Autodesk Inventor part; units mm, degrees
ref_plane "РабПлоскость1" through (-7.5, 3, -10) normal (0, 0, -1) x (-1, 0, 0)
ref_plane "YZ Plane" through (0, 0, 0) normal (1, 0, 0) x (0, 1, 0)
ref_plane "XZ Plane" through (0, 0, 0) normal (0, 1, 0) x (-1, 0, 0)
sketch "Эскиз1" plane through (0, 0, 0) normal (0, 1, 0) x (-1, 0, 0)
  line L0 (-7.5, 14.5) -> (7.5, 14.5)
  line L1 (7.5, 14.5) -> (7.5, -14.5)
  line L2 (7.5, -14.5) -> (-7.5, -14.5)
  line L3 (-7.5, -14.5) -> (-7.5, 14.5)
  line L4 (-7.5, 14.5) -> (7.5, -14.5) construction
  line L5 (7.5, 14.5) -> (-7.5, -14.5) construction
  point P0 (0, 0)
  dimension "d0" = 15
  dimension "d1" = 29
extrude "Выдавливание1" add sketch "Эскиз1" along normal blind 27
sketch "Эскиз2" plane through (0, 0, 0) normal (0, -1, 0) x (1, 0, 0)
  line L0 (12.5, 19.5) -> (-12.5, 19.5)
  line L1 (-12.5, 19.5) -> (-12.5, -15.5)
  line L2 (-12.5, -15.5) -> (12.5, -15.5)
  line L3 (12.5, -15.5) -> (12.5, 19.5)
  line L4 (7.5, 14.5) -> (7.5, -14.5)
  line L5 (-7.5, 14.5) -> (7.5, 14.5)
  point P0 (0, 0)
  dimension "d4" = 25
  dimension "d5" = 35
  dimension "d6" = 5
  dimension "d7" = 5
extrude "Выдавливание2" add sketch "Эскиз2" along normal blind 3.5
fillet "Сопряжение1" radius 1 1 edges at (-12.5, -1.75, 19.5)
fillet "Сопряжение2" radius 1 2 edges at (12.5, -1.75, 19.5) (12.5, -1.75, -15.5)
fillet "Сопряжение3" radius 1 1 edges at (-12.5, -1.75, -15.5)
sketch "Эскиз3" plane through (7.5, 27, 14.5) normal (1, 0, 0) x (0, 0, -1)
  line L0 (14.2, 0) -> (14.2, -20.2)
  line L1 (0, -27) -> (0, 0)
  line L2 (0, 0) -> (29, 0)
  line L3 (29, -27) -> (-4, -27)
  line L4 (-4, -27) -> (29, -27)
  line L5 (18.4, -27) -> (18.4, -24)
  line L6 (18.4, -24) -> (29, -24)
  line L7 (29, -27) -> (29, 0)
  line L8 (29, 0) -> (0, 0)
  line L9 (19.6, 0) -> (19.6, -15.6)
  line L10 (19.6, -15.6) -> (29, -21.4)
  line L11 (0, -25.2) -> (9.2, -25.2)
  line L12 (9.2, -25.2) -> (14.2, -20.2)
  point P0 (14.5, -27)
  dimension "d17" = 3
  dimension "d18" = 9.4
  dimension "d43" = 5
extrude "Выдавливание3" cut sketch "Эскиз3" against normal blind 23 contours L0 L12 L11 L1 L2 | L2 L7 L10 L9 | L5 L6 L7 L3
sketch "Эскиз5" plane through (0, 27, 0) normal (0, 1, 0) x (1, 0, 0)
  line L0 (-7.5, 3.9) -> (-7.5, -14.5)
  line L1 (7.5, -14.5) -> (7.5, 3.9)
  arc A0 (-7.5, 2.5) -> (7.5, 2.5) centre (0, 11.1446) ccw
  line L2 (-7.5, -0.3) -> (7.5, -0.3)
  line L3 (7.5, 5.1) -> (-7.5, 5.1)
  point P0 (0, 0)
  point P1 (0, -0.3)
  dimension "d23" = 2.6
  dimension "d24" = 2.6
extrude "Выдавливание4" cut sketch "Эскиз5" against normal blind 15.6
sketch "Эскиз6" plane through (7.5, 11.4, -5.1) normal (0, 0, -1) x (-1, 0, 0)
  line L0 (0, 0) -> (0, 15.6)
  line L1 (0, 15.6) -> (15, 15.6)
  line L2 (0, 14.2) -> (1.2, 14.2)
  line L3 (1.2, 14.2) -> (1.2, 0)
  line L4 (1.2, 0) -> (0, 0)
  line L5 (0, 0) -> (0, 14.2)
  line L6 (15, 0) -> (15, 15.6)
  line L7 (13.8, 14.2) -> (13.8, 0)
  line L8 (13.8, 0) -> (15, 0)
  line L9 (0, 14.2) -> (1.2, 14.2)
  line L10 (13.8, 14.2) -> (15.1024, 14.2)
  point P0 (7.5, -11.4)
  point P1 (15, 14.2)
  dimension "d28" = 1.2
extrude "Выдавливание5" cut sketch "Эскиз6" against normal blind 16
sketch "Эскиз7" plane through (7.5, 3, -14.5) normal (0, -1, 0) x (1, 0, 0)
  line L0 (0, 0) -> (0, 9.4)
  line L1 (0, 4.5) -> (-15, 4.5)
  line L2 (-15, 0) -> (-15, 10.6)
  line L3 (0, 0) -> (-15, 0)
  point P0 (-7.5, 14.5)
  dimension "d36" = 4.5
ref_plane "РабПлоскость1" through (-7.5, 3, -10) normal (0, 0, -1) x (-1, 0, 0)
sketch "Эскиз8" plane through (-7.5, 3, -10) normal (0, 0, -1) x (-1, 0, 0)
  line L0 (-15, 0) -> (0, 0)
  arc A0 (-7.5, -1) -> (-6, 0) centre (-7.5, 0.625) ccw
  line L1 (-15, 0) -> (0, 0)
  line L2 (-7.5, 0) -> (-7.5, -1.5688)
  point P0 (-7.5, -3)
  point P1 (-9, 0)
revolve "Вращение2" add sketch "Эскиз8" angle 360 about axis through (0, 3, -10) along (0, -1, 0)
properties part number "stopper"
Read the model definition and answer for the solid it produces. Units are mm, in the model's axes. A direction names the side the tool comes from. Coordinates: 2 decimals unless noted, no trailing zeros. Loops run counter-clockwise (first coordinate to the right, second up) from the corner with the lowest first, then second, coordinate; pieces in that order, holes last.
Q1. The part is cut by section A-A on z = -11. Write down the section's boundary in (x, y) (3 decimals), and give its area (3 significant figures).
Q2. Consider probe 1 along Y at (x, z) = (-1.5, -4); probe 2 along X at (y, z) = (5.5, -0.5); probe 3 along Y at (x, z) = (4, 10). Determine where each line is inside the solid, lowest interval first.
Q3. Each of these flat-tipped pins is pushed along its axis until it touches: pin 1 Ø4 at (x, y) = (0, 3.5) entering from -Z; pin 2 Ø7.5 at (x, z) = (-4, 3) entering from +Y; pin 3 Ø1 at (y, z) = (13.5, -4) entering from +X; pin 4 Ø4 at (y, z) = (21, -8) entering from -X. Where does it stop, or does it pass through?
Q4. The part is cut by section C-C on z = -3. Write down the section's boundary in (x, y), and give its area (3 significant figures).
Q5. Which of the six approach directions +Z, -Z, +X, -X, +Y, -Y give full straight-line access (tool end or side, diameter ignored) to faces 4 (the face through (-0.1, 19.3, 0.3)), 5 (the face through (-6, 11.4, -1)), 6 (the face through (7, 25.6, -4))?
Q6. The mould has two halves that part along Y. Classify faces 1 (the face through (6.3, 19, -3)), 2 (the face through (12.199, -1.774, -15.215)), 3 (the face through (0.1, 4.3, 2.8)): +Y half, -Y half, draft (parallel to the pull), parting line (faces both ways), or undercut.
Q7. The part is cut by section B-B on x = -3.5. Write down the section's boundary in (y, z).
Q8. The part is cut by section D-D on y = 23. Write down the section's boundary in (x, z), and give its area (3 significant figures).
Results below:
1. outline: (-12.5, -3.5) - (12.5, -3.5) - (12.5, 0) - (-12.5, 0) - close; (-7.5, 3) - (-1.118, 3) arc R1.281 ccw to (1.118, 3) - (7.5, 3) - (7.5, 7.76) - (-7.5, 7.76) - close
1. area: 160 mm2
2. probe 1: y = -3.5 to 0, 3 to 27
2. probe 2: x = -7.5 to 7.5
2. probe 3: y = -3.5 to 1.8
3. pin 1: stops at z = -14.5
3. pin 2: stops at y = 27
3. pin 3: stops at x = 6.3
3. pin 4: passes through
4. outline: (-12.5, -3.5) - (12.5, -3.5) - (12.5, 0) - (7.5, 0) - (7.5, 11.4) - (6.3, 11.4) - (6.3, 25.6) - (7.5, 25.6) - (7.5, 27) - (-7.5, 27) - (-7.5, 25.6) - (-6.3, 25.6) - (-6.3, 11.4) - (-7.5, 11.4) - (-7.5, 0) - (-12.5, 0) - close
4. area: 458 mm2
5. face 4: +Z, +Y
5. face 5: +Z, -X
5. face 6: +Z, -Z, +X
6. face 1: undercut
6. face 2: draft
6. face 3: +Y half
7. outline: (-3.5, -15.5) - (0, -15.5) - (0, -3.9) - (3, -3.9) - (3, -14.5) - (5.6, -14.5) - (11.4, -5.1) - (27, -5.1) - (27, -0.25) - (11.4, -0.25) - (11.4, 0.3) - (6.8, 0.3) - (1.8, 5.3) - (1.8, 14.5) - (0, 14.5) - (0, 19.5) - (-3.5, 19.5) - close
8. outline: (-6.3, -5.1) - (6.3, -5.1) - (6.3, -1.59) arc R11.44 ccw to (-6.3, -1.59) - close
8. area: 60.4 mm2
